For this review, take the finished solid that the model builds, in its own axes (mm). Face numbers are marked on the shaded views. A direction names the side the tool comes from. Round coordinates to 2 decimals unless told otherwise and drop trailing zeros. Write each loop counter-clockwise with the first axis right and the second up, starting at its lowest first coordinate (ties: lowest second). Pieces come first, ordered by that corner, then holes.
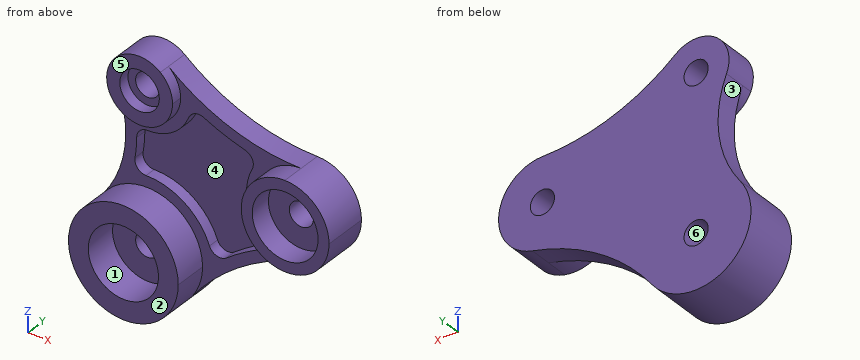
from build123d import *

# Parameters (mm, degrees)
F1_DEPTH  = 10
F2_DEPTH  = 15
F3_DEPTH  = 25
F4_DEPTH  = 20
F5_R      = 16
F5_R_2    = 9
F5_R_3    = 15
F6_DEPTH  = 15
F7_R      = 5.5
F8_DEPTH  = 10.001
F10_DEPTH = 5
F11_R     = 5


with BuildPart() as f1:
    # F0 (on Front) → F1 (new body)
    with BuildSketch(Plane.XZ):
        with BuildLine():
            ThreePointArc((-20, 15), (7.905694, 23.717082), (25, 0))
            ThreePointArc((25, 0), (23.736535, -7.847096), (20.073847, -14.901029))
            ThreePointArc((20.073847, -14.901029), (44.154845, 7.848858), (74.583385, 20.946787))
            ThreePointArc((74.583385, 20.946787), (50.140462, 38.048353), (69.881043, 60.414165))
            ThreePointArc((69.881043, 60.414165), (37.823204, 65.784342), (9.452181, 81.647157))
            ThreePointArc((9.452181, 81.647157), (13.542207, 76.450476), (15, 70))
            ThreePointArc((15, 70), (2.941742, 55.29129), (-13.846154, 64.230769))
            ThreePointArc((-13.846154, 64.230769), (-10.386106, 38.798263), (-20, 15))
        make_face()
    extrude(amount=F1_DEPTH)

    # F0 (on Front) → F2 (join)
    with BuildSketch(Plane.XZ):
        with BuildLine():
            ThreePointArc((9.452181, 81.647157), (-8.981057, 82.014184), (-13.846154, 64.230769))
            ThreePointArc((-13.846154, 64.230769), (2.941742, 55.29129), (15, 70))
            ThreePointArc((15, 70), (13.542207, 76.450476), (9.452181, 81.647157))
        make_face()
    extrude(amount=F2_DEPTH)

    # F0 (on Front) → F3 (join)
    with BuildSketch(Plane.XZ):
        with BuildLine():
            ThreePointArc((20.073847, -14.901029), (23.736535, -7.847096), (25, 0))
            ThreePointArc((25, 0), (7.905694, 23.717082), (-20, 15))
            ThreePointArc((-20, 15), (-14.95056, -20.036985), (20.073847, -14.901029))
        make_face()
    extrude(amount=F3_DEPTH)

    # F0 (on Front) → F4 (join)
    with BuildSketch(Plane.XZ):
        with BuildLine():
            ThreePointArc((69.881043, 60.414165), (50.140462, 38.048353), (74.583385, 20.946787))
            ThreePointArc((74.583385, 20.946787), (85.67909, 27.998153), (90, 40.414519))
            ThreePointArc((90, 40.414519), (84.100015, 54.59865), (69.881043, 60.414165))
        make_face()
    extrude(amount=F4_DEPTH)

    # F5 (on face) → F6 (cut)
    with BuildSketch(Plane.XZ.offset(25)):
        Circle(F5_R)
        with Locations((0, 70)):
            Circle(F5_R_2)
        with Locations((70, 40.414519)):
            Circle(F5_R_3)
    extrude(amount=-F6_DEPTH, mode=Mode.SUBTRACT)

    # F7 (on face) → F8 (cut, through all)
    with BuildSketch(Plane.XZ.offset(10)):
        Circle(F7_R)
        with Locations((0, 70)):
            Circle(F7_R)
        with Locations((70, 40.414519)):
            Circle(F7_R)
    extrude(amount=-F8_DEPTH, mode=Mode.SUBTRACT)

    # F9 (on face) → F10 (cut)
    with BuildSketch(Plane.XZ.offset(10)):
        with BuildLine():
            ThreePointArc((51.331935, 57.042909), (35.156253, 61.427848), (19.940051, 68.452632))
            ThreePointArc((19.940051, 68.452632), (11.500487, 53.637274), (-5.297662, 50.714389))
            ThreePointArc((-5.297662, 50.714389), (-5.246639, 39.797168), (-7.352958, 29.084945))
            ThreePointArc((-7.352958, 29.084945), (17.164465, 24.604494), (29.835004, 3.142063))
            ThreePointArc((29.835004, 3.142063), (42.1494, 12.509642), (55.761443, 19.865468))
            ThreePointArc((55.761443, 19.865468), (45.175577, 37.456812), (51.331935, 57.042909))
        make_face()
    extrude(amount=-F10_DEPTH, mode=Mode.SUBTRACT)

    # F11
    f11_edges = [f1.edges().sort_by_distance(p)[0] for p in [
        (19.940051, -7.5, 68.452632),
        (-5.297662, -7.5, 50.714389),
        (51.331935, -7.5, 57.042909),
        (55.761443, -7.5, 19.865468),
        (-7.352958, -7.5, 29.084945),
        (29.835004, -7.5, 3.142063),
    ]]
    fillet(f11_edges, radius=F11_R)


solid = f1.part
(1) For the marked faces 4, 5 and 6, list the 3-axis set-ups (+Z, -Z, +X, -X, +Y, -Y) from which the entire face can be reached by the end or side of a thin tool; tool diameter is ignored.
Geometry check:
face 4: -Y
face 5: +Z, -X, -Y
face 6: +Y, -Y
(2) For line 1 along Z through (x, y) = (0, -13); line 2 along Z through (x, y) = (2, -13.75); line 3 along X through (y, z) = (-11.75, 45), list the stretches that pass through material, from the lowest coordinate up.
Geometry check:
line 1: z = -25 to -16, 16 to 25, 55 to 61, 79 to 85
line 2: z = -24.92 to -15.87, 15.87 to 24.92, 55.13 to 61.23, 78.77 to 84.87
line 3: x = 50.53 to 55.72, 84.28 to 89.47
(3) We need section A-A, the plane z = -10. Give the boundary of the cut face in (x, y).
Geometry check:
outline: (-22.91, -25) - (-12.49, -25) - (-12.49, -10) - (12.49, -10) - (12.49, -25) - (22.91, -25) - (22.91, -10) - (23.97, -10) - (23.97, 0) - (-22.91, 0) - close
(4) For pin 1 Ø8 at (x, y) = (54, -19) entering from +Z; pin 2 Ø14.5 at (x, z) = (-1, 74.5) entering from -Y; pin 3 Ø9 at (x, z) = (0, 0) entering from +Y; pin 4 Ø12 at (x, y) = (65.5, -15.5) entering from +Z, all flat-tipped, find the tip position at first contact; note any pin that passes through.
Geometry check:
pin 1: stops at z = 56.41
pin 2: stops at y = -15
pin 3: passes through
pin 4: stops at z = 60.62
(5) We need section B-B, the plane y = -8.5. State how many separate pieces and enclosed holes the cut face has, and give its area (3 significant figures).
Geometry check:
separate pieces: 1
enclosed holes: 4
area: 5,030 mm2
(6) Mouldability with a two-part tool opening along X and no side actions: class the marked faces 1, 2 and 3 as pulls with the +X half, pulls with the -X half, needs draft (parallel to the pull), parting line crosses it, or undercut.
Geometry check:
face 1: undercut
face 2: needs draft
face 3: pulls with the -X half
